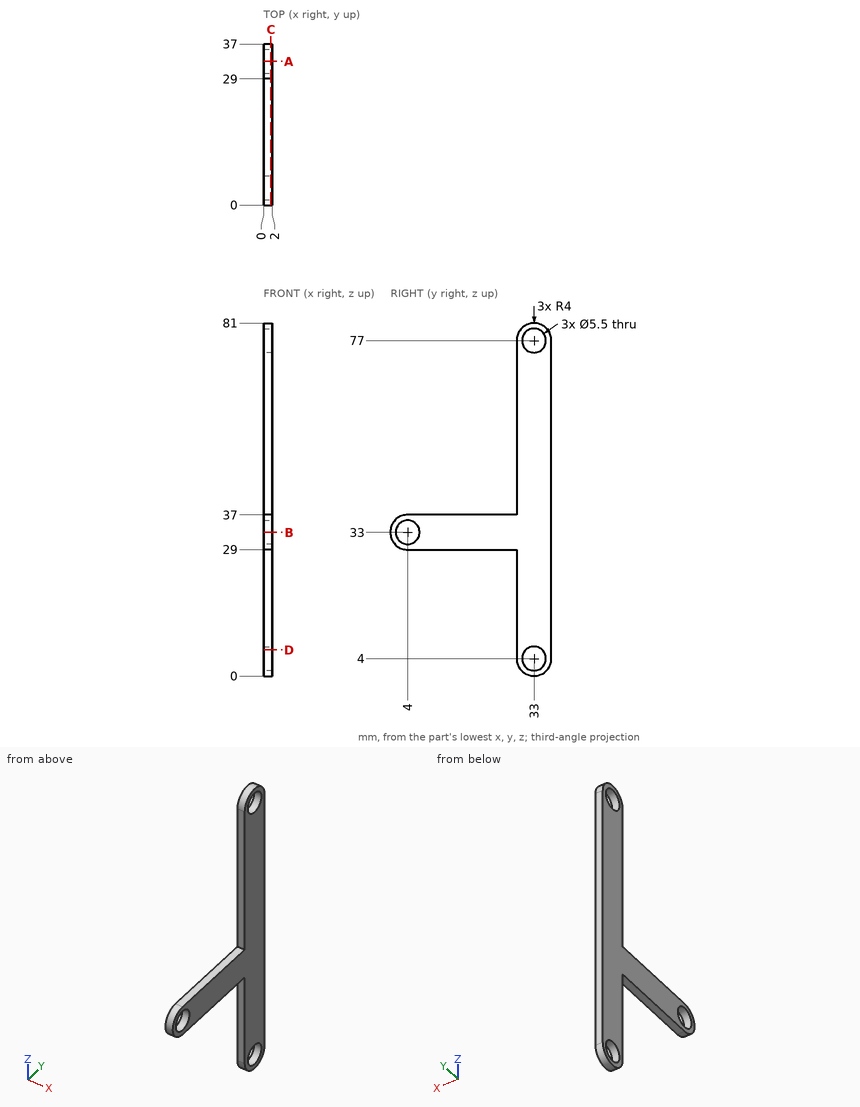
Source: three-view drawing plus pictorial views. Frame: mm from the lowest corner of the part. Give positions to 0.01 mm unless a question says otherwise; leave off trailing zeros. Loops run counter-clockwise (first coordinate to the right, second up) from the corner with the lowest first, then second, coordinate; pieces in that order, holes last. Notation, with made-up numbers: (-27.75, -21.5) -> (17.25, -21.5) arc R31 cw to (17.25, 16.5) -> close; hole circle Ø8 at (-15, -29.5). An arc over 180 degrees is marked (long way). Put each result on its own line as item: value. Start each with the question number.
1) Cut plane C-C (x = 1.7). Return loops of the section in (y, z), then the cut area to 3 significant figures.
2) Cut plane B-B (z = 33). Return loops of the section in (x, y).
3) Material intervals for probe 1 along Y at (x, z) = (0.95, 77); probe 2 along Z at (x, y) = (0.15, 13), sorted ascending.
4) Cut plane A-A (y = 33). Return loops of the section in (x, z), then the cut area to 3 significant figures.
5) Cut plane D-D (z = 6). Return loops of the section in (x, y).
Results are:
1. outline: (4, 29) -> (29, 29) -> (29, 4) arc R4 ccw to (37, 4) -> (37, 77) arc R4 ccw to (29, 77) -> (29, 37) -> (4, 37) arc R4 ccw to start; hole circle Ø5.5 at (4, 33); hole circle Ø5.5 at (33, 4); hole circle Ø5.5 at (33, 77)
1. area: 788 mm2
2. outline: (0, 0) -> (2, 0) -> (2, 1.25) -> (0, 1.25) -> close; (0, 6.75) -> (2, 6.75) -> (2, 37) -> (0, 37) -> close
3. probe 1: y = 29 to 30.25, 35.75 to 37
3. probe 2: z = 29 to 37
4. outline: (0, 0) -> (2, 0) -> (2, 1.25) -> (0, 1.25) -> close; (0, 6.75) -> (2, 6.75) -> (2, 74.25) -> (0, 74.25) -> close; (0, 79.75) -> (2, 79.75) -> (2, 81) -> (0, 81) -> close
4. area: 140 mm2
5. outline: (0, 29) -> (2, 29) -> (2, 31.11) -> (0, 31.11) -> close; (0, 34.89) -> (2, 34.89) -> (2, 37) -> (0, 37) -> close
